from build123d import *

# Parameters (mm, degrees)
FILLET1_R = 1
SKETCH3_W = 1.25
SKETCH3_H = 8.5


with BuildPart() as part:
    # Sketch1 → Revolve1 (revolve)
    with BuildSketch(Plane.XY):
        Polygon((-8.5, -6.35), (-8.5, 0), (-15, 0), (-15, 1.5), (-13.5, 1.5), (-13.5, 13.5), (-15, 13.5), (-15, 15), (0, 15), (0, 7.65), (-4, 7.65), (-4, -6.35), align=None)
    revolve(axis=Axis((0, 15, 0), (0, -1, 0)))

    # Fillet1
    fillet1_edges = [part.edges().sort_by_distance(p)[0] for p in [
        (8.5, -6.35, 0),
        (4, -6.35, 0),
    ]]
    fillet(fillet1_edges, radius=FILLET1_R)

    # Sketch3 → M3x0.5 Tapped Hole1 (revolve, cut)
    with BuildSketch(Plane(origin=(0, -2.35, 0), x_dir=(0, 1, 0), z_dir=(1, 0, 0))):
        with Locations((0.625, 4.25)):
            Rectangle(SKETCH3_W, SKETCH3_H)
    revolve(axis=Axis((0, -2.35, -6.35), (0, 0, 1)), mode=Mode.SUBTRACT)


solid = part.part
Source: CAD feature listing. Evaluate the final solid. Frame: model axes, mm. A direction names the side the tool comes from. Coordinates: 2 decimals unless noted, no trailing zeros. Order: outer loops, then holes, each group sorted by start corner. A loop starts at its lowest first (then second) coordinate and runs counter-clockwise, first axis right, second up. Notation, with made-up numbers: M 84,0 L 95,0 A6 cw 95,7 Z; hole C 62,-6.75 d2. An arc over 180 degrees is marked long. Write each question's results on one line, items separated by ' | '. Start each with the question number.
1. Section C-C, the plane y = 7. Return the cut outline in (x, z).
2. Material intervals for L1, parallel to Z at x = 0, y = 0.5; L2, parallel to Y at x = 0, z = 6.05; L3, parallel to Y at x = 13.5, z = 2, sorted ascending.
3. Reachability of faces 1 (the face through (14.985, 0.76, -0.66)), 2 (the face through (-0.38, -1.16, 6.18)), 3 (the face through (2.93, 7.58, 13.18)), 4 (the face through (6.5, 0, 6.5)) from +Z, -Z, +X, -X, +Y, -Y: full face, straight path, thin tool, end or side. Return the list, or none.
4. Draft query along X for faces 5 (the face through (-4.57, -2.638, -7.167)), 6 (the face through (-11.18, 13.5, -7.85)), 7 (the face through (0, 7.65, 0)). Return one class per face: +X half, -X half, draft (parallel to the pull), parting line (faces both ways), or undercut.
5. Section D-D, the plane x = 9. Return the cut outline in (y, z).
6. Section B-B, the plane z = 0. Return the cut outline in (x, y).
7. Section A-A, the plane x = 0. Return the cut outline in (y, z).
8. Pin query (flat end, axial travel): pin 1 (1.5 mm diameter, centred on x = -8.5, y = 5.5, fed in from -Z); pin 2 (3 mm diameter, centred on x = 9.5, z = -8, fed in from -Y); pin 3 (4 mm diameter, centred on x = -8.5, y = 5, fed in from +Z). Return the tip coordinate at first contact, or that it passes through.
Solution:
1) outline: C 0,0 d27; hole C 0,0 d8
2) L1: -15 to -4, 4 to 15 | L2: -6.35 to -3.6, -1.1 to 15 | L3: 0 to 1.5, 13.5 to 15
3) face 1: +Y, -Y | face 2: +Z | face 3: none | face 4: -Y
4) face 5: parting line | face 6: draft | face 7: undercut
5) outline: M 0,-12 L 1.5,-12 L 1.5,-10.06 L 13.5,-10.06 L 13.5,-12 L 15,-12 L 15,12 L 13.5,12 L 13.5,10.06 L 1.5,10.06 L 1.5,12 L 0,12 Z
6) outline: M -15,0 L -8.5,0 L -8.5,-5.35 A1 ccw -7.5,-6.35 L -5,-6.35 A1 ccw -4,-5.35 L -4,7.65 L 4,7.65 L 4,-5.35 A1 ccw 5,-6.35 L 7.5,-6.35 A1 ccw 8.5,-5.35 L 8.5,0 L 15,0 L 15,1.5 L 13.5,1.5 L 13.5,13.5 L 15,13.5 L 15,15 L -15,15 L -15,13.5 L -13.5,13.5 L -13.5,1.5 L -15,1.5 Z
7) outline: M -6.35,-7.5 A1 ccw -5.35,-8.5 L 0,-8.5 L 0,-15 L 1.5,-15 L 1.5,-13.5 L 13.5,-13.5 L 13.5,-15 L 15,-15 L 15,15 L 13.5,15 L 13.5,13.5 L 1.5,13.5 L 1.5,15 L 0,15 L 0,8.5 L -1.1,8.5 L -1.1,4 L 7.65,4 L 7.65,-4 L -5.35,-4 A1 ccw -6.35,-5 Z; M -6.35,5 A1 ccw -5.35,4 L -3.6,4 L -3.6,8.5 L -5.35,8.5 A1 ccw -6.35,7.5 Z
8) pin 1: z = -11.05 | pin 2: y = 0 | pin 3: z = 11.83
